Design review of the part built by this model. Coordinates are the model's own, in mm. A direction names the side the tool comes from. Coordinates: 2 decimals unless noted, no trailing zeros. Write each loop counter-clockwise with the first axis right and the second up, starting at its lowest first coordinate (ties: lowest second). Pieces come first, ordered by that corner, then holes.
Q1. Take a section at B-B, the plane z = 3.4. Write out the cut boundary in (x, y) (3 decimals).
Q2. For pin 1 Ø22 at (x, y) = (-29.5, -3) entering from +Z; pin 2 Ø0.9 at (y, z) = (15.5, 3) entering from +X; pin 3 Ø0.7 at (y, z) = (28, 5.5) entering from +X, all flat-tipped, find the tip position at first contact; note any pin that passes through.
Q3. Take a section at D-D, the plane x = -130. Write out the cut boundary in (y, z) (3 decimals), plus the area to 3 significant figures.
Q4. For L1, parallel to Y at x = -77.5, z = 2.25 (3 decimals); L2, parallel to Y at x = -126.5, z = 5.4 (3 decimals); L3, parallel to Z at x = -83, y = 3, list the stretches that pass through material, from the lowest coordinate up.
Q5. The part is to be moulded in two halves that separate along Y. For faces 1 (the flat face through (-82, 1, 0)), 2 (the flat face through (-79, 36.125, 3)), 3 (the flat face through (-72, -10, 3)), say which applies: released by +Y, released by -Y, zero draft, split by the parting line, or undercut.
Q6. Take a section at A-A, the plane x = -65. Write out the cut boundary in (y, z) (3 decimals), plus the area to 3 significant figures.
Q7. Take a section at C-C, the plane y = 4. Write out the cut boundary in (x, z).
Q8. For faces 4 (the flat face through (-34, 29, 4.35)), 5 (the flat face through (-18.346, -29, 2)), 6 (the flat face through (-91, 0, 5.5)), 7 (the cylindrical face through (-141.92, 34.62, 2.86)), 8 (the flat face through (-72, 10, 3)), list the 3-axis set-ups (+Z, -Z, +X, -X, +Y, -Y) from which the entire face can be reached by the end or side of a thin tool; tool diameter is ignored.
from build123d import *

# Parameters (mm, degrees)
F0_W      = 210
F0_H      = 52.25
F0_W_2    = 200
F0_H_2    = 42.25
F1_DEPTH  = 5.5
F0_W_3    = 230
F0_H_3    = 72.25
F2_DEPTH  = 5.65
F4_DEPTH  = 100
F6_DEPTH  = 5
F7_SIZE   = 1.75
F8_R      = 5
F9_R      = 5
F10_W     = 20
F10_H     = 5.5
F11_DEPTH = 110
F12_W     = 30
F12_H     = 1.15
F13_DEPTH = 25
F14_R     = 5


with BuildPart() as f1:
    # F0 (on Top) → F1 (new body)
    with BuildSketch(Plane.XY):
        with Locations((-28.3456140757, 0)):
            Rectangle(F0_W, F0_H)
        with Locations((-28.3456140757, 0)):
            Rectangle(F0_W_2, F0_H_2, mode=Mode.SUBTRACT)
    extrude(amount=F1_DEPTH)

    # F0 (on Top) → F2 (join)
    with BuildSketch(Plane.XY):
        with Locations((-28.3456140757, 0)):
            Rectangle(F0_W_3, F0_H_3)
        with Locations((-28.3456140757, 0)):
            Rectangle(F0_W, F0_H, mode=Mode.SUBTRACT)
    extrude(amount=F2_DEPTH)

    # F3 (on face) → F4 (cut)
    with BuildSketch(Plane.XZ.offset(36.125)):
        Polygon((-48.3456140757, 5.65), (-48.3456140757, 4.35), (-18.3456140757, 4.35), (-18.3456140757, 0), (86.6543859243, 0), (86.6543859243, 5.65), align=None)
    extrude(amount=-F4_DEPTH, mode=Mode.SUBTRACT)

    # F5 (on face) → F6 (cut)
    with BuildSketch(Plane.XY.offset(5.65)):
        with BuildLine():
            ThreePointArc((-135.231653045, 29.7610389693), (-136.3119570383, 31.3778281512), (-138.2190899121, 30.9984758364))
            Line((-138.2190899121, 30.9984758364), (-135.7442161779, 28.5236021022))
            ThreePointArc((-135.7442161779, 28.5236021022), (-135.3648638631, 29.0913429627), (-135.231653045, 29.7610389693))
        make_face()
        with BuildLine():
            Line((-135.7442161779, 28.5236021022), (-138.2190899121, 30.9984758364))
            ThreePointArc((-138.2190899121, 30.9984758364), (-138.2190899121, 28.5236021022), (-135.7442161779, 28.5236021022))
        make_face()
        with BuildLine():
            ThreePointArc((-135.7442161779, -28.5236021022), (-138.2190899121, -28.5236021022), (-138.2190899121, -30.9984758364))
            Line((-138.2190899121, -30.9984758364), (-135.7442161779, -28.5236021022))
        make_face()
        with BuildLine():
            Line((-135.7442161779, -28.5236021022), (-138.2190899121, -30.9984758364))
            ThreePointArc((-138.2190899121, -30.9984758364), (-136.3119570383, -31.3778281512), (-135.231653045, -29.7610389693))
            ThreePointArc((-135.231653045, -29.7610389693), (-135.3648638631, -29.0913429627), (-135.7442161779, -28.5236021022))
        make_face()
    extrude(amount=-F6_DEPTH, mode=Mode.SUBTRACT)

    # F7
    f7_edges = [f1.edges().sort_by_distance(p)[0] for p in [
        (-135.744216, -28.523602, 0.65),
        (-138.731653, 29.761039, 0.65),
    ]]
    chamfer(f7_edges, length=F7_SIZE)

    # F8
    f8_edges = [f1.edges().sort_by_distance(p)[0] for p in [
        (-143.345614, 36.125, 2.825),
        (-143.345614, -36.125, 2.825),
    ]]
    fillet(f8_edges, radius=F8_R)

    # F9
    f9_edges = [f1.edges().sort_by_distance(p)[0] for p in [
        (-128.345614, -21.125, 2.75),
        (-128.345614, 21.125, 2.75),
    ]]
    fillet(f9_edges, radius=F9_R)

    # F10 (on face) → F11 (join)
    with BuildSketch(Plane.YZ.offset(-128.3456140757)):
        with Locations((0, 2.75)):
            Rectangle(F10_W, F10_H)
    extrude(amount=F11_DEPTH)

    # F12 (on face) → F13 (cut)
    with BuildSketch(Plane.XZ.offset(10)):
        with Locations((-33.3456140757, 4.925)):
            Rectangle(F12_W, F12_H)
    extrude(amount=-F13_DEPTH, mode=Mode.SUBTRACT)

    # F14
    f14_edges = [f1.edges().sort_by_distance(p)[0] for p in [
        (-128.345614, -10, 2.75),
        (-128.345614, 10, 2.75),
    ]]
    fillet(f14_edges, radius=F14_R)


solid = f1.part
Responses:
1. outline: (-143.346, -31.125) arc R5 ccw to (-138.346, -36.125) - (-18.346, -36.125) - (-18.346, -21.125) - (-123.346, -21.125) arc R5 cw to (-128.346, -16.125) - (-128.346, -15) arc R5 cw to (-123.346, -10) - (-18.346, -10) - (-18.346, 10) - (-123.346, 10) arc R5 cw to (-128.346, 15) - (-128.346, 16.125) arc R5 cw to (-123.346, 21.125) - (-18.346, 21.125) - (-18.346, 36.125) - (-138.346, 36.125) arc R5 ccw to (-143.346, 31.125) - close; hole circle Ø3.5 at (-136.982, -29.761); hole circle Ø3.5 at (-136.982, 29.761)
2. pin 1: stops at z = 4.35
2. pin 2: stops at x = -128.35
2. pin 3: stops at x = -48.35
3. outline: (-36.125, 0) - (36.125, 0) - (36.125, 5.65) - (26.125, 5.65) - (26.125, 5.5) - (-26.125, 5.5) - (-26.125, 5.65) - (-36.125, 5.65) - close
3. area: 400 mm2
4. L1: y = -36.125 to -21.125, -10 to 10, 21.125 to 36.125
4. L2: y = -36.125 to -20.004, -11.121 to 11.121, 20.004 to 36.125
4. L3: z = 0 to 5.5
5. face 1: zero draft
5. face 2: released by +Y
5. face 3: undercut
6. outline: (-36.125, 0) - (-21.125, 0) - (-21.125, 5.5) - (-26.125, 5.5) - (-26.125, 5.65) - (-36.125, 5.65) - close; (-10, 0) - (10, 0) - (10, 5.5) - (-10, 5.5) - close; (21.125, 0) - (36.125, 0) - (36.125, 5.65) - (26.125, 5.65) - (26.125, 5.5) - (21.125, 5.5) - close
6. area: 278 mm2
7. outline: (-143.35, 0) - (-18.35, 0) - (-18.35, 4.35) - (-48.35, 4.35) - (-48.35, 5.5) - (-133.35, 5.5) - (-133.35, 5.65) - (-143.35, 5.65) - close
8. face 4: +Z, +X, +Y, -Y
8. face 5: +Z, -Z, +X, +Y, -Y
8. face 6: +Z, +X
8. face 7: +Z, -Z, -X, +Y
8. face 8: +Z, -Z, +X
